For this review, take the finished solid that the model builds, in its own axes (mm). A direction names the side the tool comes from. Round coordinates to 2 decimals unless told otherwise and drop trailing zeros. Write each loop counter-clockwise with the first axis right and the second up, starting at its lowest first coordinate (ties: lowest second). Pieces come first, ordered by that corner, then holes. Notation, with made-up numbers: M -22.75,-23 L -0.75,-23 A24 cw -0.75,10 Z; hole C 11,38.5 d4. An arc over 180 degrees is marked long. Use one line per item in the form item = value. Start each with the question number.
Item 1: For P1, Ø3.5, axis at x = 65, y = 2.5, coming from the +Z side; P2, Ø3, axis at x = 17, z = -44, coming from the +Y side; P3, Ø10, axis at x = 127, z = -20, coming from the +Y side; P4, Ø6, axis at y = 14, z = -41.5, coming from the -X side, all flat-tipped, find the tip position at first contact; note any pin that passes through.
Item 2: For line 1 (Y direction, x = -20, z = -15); line 2 (X direction, y = 13, z = -8.5); line 3 (Y direction, x = 164.5, z = -49.5), list the stretches that pass through material, from the lowest coordinate up. Write a range as [from, to].
Item 3: Draft analysis for pull direction Y (two halves, no side actions). For faces 5 (the flat face through (84.13, 10.5, -50.09)), 6 (the flat face through (6.08, 2, -47.45)), 7 (the flat face through (157.48, 4, -10)), state which applies: released by +Y, released by -Y, zero draft, split by the parting line, or undercut.
Item 4: Add section D-D (z = -59). State the section outline as (x, y) points, and give its area (3 significant figures).
Item 5: For faces 1 (the flat face through (-35.262, 6.068, -19.775)), 2 (the cylindrical face through (176.8, 3.96, -44.44)), 3 (the flat face through (64, 2, -5.3)), 4 (the flat face through (-35.13, 6.07, -37.5)), list the 3-axis set-ups (+Z, -Z, +X, -X, +Y, -Y) from which the entire face can be reached by the end or side of a thin tool; tool diameter is ignored.
Item 6: Add section B-B (x = 98). State the section outline as (y, z) points.
Item 7: Add section A-A (x = 163.5). State the section outline as (y, z) points.
Item 8: Add section C-C (y = 13.5). State the section outline as (x, z) points, and give its area (3 significant figures).
from build123d import *

# Parameters (mm, degrees)
BOSS_EXTRUDE1_DEPTH = 195.58
SKETCH2_R           = 3.3147
CUT_EXTRUDE1_DEPTH  = 38.1
SKETCH3_W           = 27.94
SKETCH3_H           = 4.064
CUT_EXTRUDE2_DEPTH  = 405.649982083
CUT_EXTRUDE3_DEPTH  = 4.064
SKETCH5_W           = 101.6
SKETCH5_H           = 20.32
CUT_EXTRUDE4_DEPTH  = 165.1
BOSS_EXTRUDE2_DEPTH = 4.064
SKETCH7_R           = 1.905
CUT_EXTRUDE5_DEPTH  = 12.7


with BuildPart() as part:
    # Sketch1 → Boss-Extrude1 (new, symmetric)
    with BuildSketch(Plane(origin=(0, 0, 0), x_dir=(0, 0, -1), z_dir=(1, 0, 0))):
        Polygon((0, 0), (0, 20.32), (101.6, 0.4), (101.6, 0), align=None)
    extrude(amount=BOSS_EXTRUDE1_DEPTH, both=True)

    # Sketch2 → Cut-Extrude1 (cut)
    with BuildSketch(Plane(origin=(195.58, 0, 0), x_dir=(0, 0, -1), z_dir=(1, 0, 0))):
        with Locations((9.652, 3.81)):
            Circle(SKETCH2_R)
        with Locations((47.752, 3.81)):
            Circle(SKETCH2_R)
    cut_extrude1 = extrude(amount=-CUT_EXTRUDE1_DEPTH, mode=Mode.SUBTRACT)

    # Mirror3: Cut-Extrude1 across plane
    add(cut_extrude1.mirror(Plane(origin=(0, 0, 0), x_dir=(0, 0, 1), z_dir=(1, 0, 0))), mode=Mode.SUBTRACT)

    # Sketch3 → Cut-Extrude2 (cut, through all)
    with BuildSketch(Plane.ZY.offset(195.58)):
        with Locations((-28.702, 2.032)):
            Rectangle(SKETCH3_W, SKETCH3_H)
    extrude(amount=-CUT_EXTRUDE2_DEPTH, mode=Mode.SUBTRACT)

    # Sketch4 → Cut-Extrude3 (cut)
    with BuildSketch(Plane.XZ):
        Polygon((5.40665728, -42.672), (-10.788895147, -42.672), (-12.114518933, -52.104303355), (6.732281067, -52.104303355), align=None)
        Polygon((139.397762134, -42.672), (123.202209707, -42.672), (121.87658592, -52.104303355), (140.72338592, -52.104303355), align=None)
        Polygon((121.87658592, -5.299696645), (123.202209707, -14.732), (139.397762134, -14.732), (140.72338592, -5.299696645), align=None)
        Polygon((-12.114518933, -5.299696645), (-10.788895147, -14.732), (5.40665728, -14.732), (6.732281067, -5.299696645), align=None)
        Polygon((72.402209707, -42.672), (56.20665728, -42.672), (54.881033493, -52.104303355), (73.727833493, -52.104303355), align=None)
        Polygon((54.881033493, -5.299696645), (56.20665728, -14.732), (72.402209707, -14.732), (73.727833493, -5.299696645), align=None)
    extrude(amount=-CUT_EXTRUDE3_DEPTH, mode=Mode.SUBTRACT)

    # Sketch5 → Cut-Extrude4 (cut)
    with BuildSketch(Plane.ZY.offset(195.58)):
        with Locations((-50.8, 10.16)):
            Rectangle(SKETCH5_W, SKETCH5_H)
    extrude(amount=-CUT_EXTRUDE4_DEPTH, mode=Mode.SUBTRACT)

    # Sketch6 → Boss-Extrude2 (add)
    with BuildSketch(Plane.XZ.offset(-4.064)):
        Polygon((-30.48, -20.447), (-30.48, -36.845752427), (-39.912303355, -38.171376213), (-39.912303355, -19.121376213), align=None)
    extrude(amount=-BOSS_EXTRUDE2_DEPTH)

    # Sketch7 → Cut-Extrude5 (cut)
    with BuildSketch(Plane.ZY.offset(30.48)):
        with Locations((-15.24, 8.128)):
            Circle(SKETCH7_R)
        with Locations((-45.72, 8.128)):
            Circle(SKETCH7_R)
    extrude(amount=-CUT_EXTRUDE5_DEPTH, mode=Mode.SUBTRACT)


solid = part.part
Calculated:
q1.P1 = 0
q1.P2 = 11.99
q1.P3 = 17.38
q1.P4 = -30.48
q2.line_1 = [4.06, 6.24], [10.02, 17.38]
q2.line_2 = [-30.48, 195.58]
q2.line_3 = [0, 0.99], [6.63, 10.61]
q3.face_5 = released by +Y
q3.face_6 = zero draft
q3.face_7 = undercut
q4.outline = M -30.48,0 L 195.58,0 L 195.58,8.75 L -30.48,8.75 Z
q4.area = 1,980 mm^2
q5.face_1 = +Z, +Y, -Y
q5.face_2 = +X
q5.face_3 = -Y
q5.face_4 = -Z, +Y, -Y
q6.outline = M 0,-101.6 L 0.4,-101.6 L 20.32,0 L 0,0 L 0,-14.73 L 4.06,-14.73 L 4.06,-42.67 L 0,-42.67 Z
q7.outline = M 0,-101.6 L 0.4,-101.6 L 20.32,0 L 0,0 L 0,-14.73 L 4.06,-14.73 L 4.06,-42.67 L 0,-42.67 Z; hole C 3.81,-47.75 d6.63; hole C 3.81,-9.65 d6.63
q8.outline = M -30.48,-34.78 L 195.58,-34.78 L 195.58,0 L -30.48,0 Z
q8.area = 7,860 mm^2
